Autodesk Inventor part; units mm, degrees
ref_plane "YZ Plane" through (0, 0, 0) normal (1, 0, 0) x (0, 1, 0)
ref_plane "XZ Plane" through (0, 0, 0) normal (0, 1, 0) x (-1, 0, 0)
ref_plane "XY Plane" through (0, 0, 0) normal (0, 0, 1) x (1, 0, 0)
sketch "Sketch1" plane through (0, 0, 0) normal (0, 0, 1) x (1, 0, 0)
  arc A0 (-16, 4) -> (-16, -4) centre (-16, 0) ccw
  arc A1 (16, -4) -> (16, 4) centre (16, 0) ccw
  line L0 (-16, -4) -> (16, -4)
  line L1 (-16, 4) -> (16, 4)
  line L2 (-28, 0) -> (28, 0)
  line L3 (0, -5.6) -> (0, 5.6)
  point P0 (0, 0)
  dimension "d3" = 4
  dimension "d4" = 4
  dimension "d5" = 32
  dimension "d6" = 32
  dimension "d7" = 0
  dimension "d8" = 16
  dimension "d9" = 32
  dimension "d10" = 32
extrude "Extrusion1" add sketch "Sketch1" along normal blind 8
sketch "Sketch2" plane through (0, 0, 8) normal (0, 0, 1) x (1, 0, 0)
  arc A0 (-16, 4) -> (-16, -4) centre (-16, 0) ccw
  circle A1 centre (-16, 0) radius 2.5
  line L0 (-28, 0) -> (28, 0)
  circle A2 centre (-8, 0) radius 2.5
  circle A3 centre (0, 0) radius 2.5
  circle A4 centre (8, 0) radius 2.5
  circle A5 centre (16, 0) radius 2.5
  dimension "d13" = 5
  dimension "d19" = 8
extrude "Extrusion2" cut sketch "Sketch2" against normal through all
sketch "Sketch3" plane through (0, 0, 8) normal (0, 0, 1) x (1, 0, 0)
  circle A0 centre (16, 0) radius 2.5
  circle A1 centre (8, 0) radius 2.5
  circle A2 centre (0, 0) radius 2.5
  circle A3 centre (-8, 0) radius 2.5
  circle A4 centre (-16, 0) radius 2.5
  arc A5 (-16, 4) -> (-16, -4) centre (-16, 0) ccw
  circle A6 centre (-16, 0) radius 3
  line L0 (-28, 0) -> (28, 0)
  circle A7 centre (-8, 0) radius 3
  circle A8 centre (0, 0) radius 3
  circle A9 centre (8, 0) radius 3
  circle A10 centre (16, 0) radius 3
  dimension "d23" = 6
  dimension "d29" = 8
extrude "Extrusion3" cut sketch "Sketch3" against normal blind 0.8 contours L0 A10 A0 | A0 L0 A10 | A6 L0 A4 | L0 A4 A6 | A7 L0 A3 | L0 A3 A7 | A8 L0 A2 | L0 A2 A8 | A9 L0 A1 | L0 A1 A9
sketch "Sketch4" plane through (0, 0, 0) normal (0, 0, -1) x (-1, 0, 0)
  circle A0 centre (-16, 0) radius 2.5
  circle A1 centre (-8, 0) radius 2.5
  circle A2 centre (0, 0) radius 2.5
  circle A3 centre (8, 0) radius 2.5
  circle A4 centre (16, 0) radius 2.5
  arc A5 (-16, 4) -> (-16, -4) centre (-16, 0) ccw
  circle A6 centre (-16, 0) radius 3
  line L0 (28, 0) -> (-28, 0)
  circle A7 centre (-8, 0) radius 3
  circle A8 centre (0, 0) radius 3
  circle A9 centre (8, 0) radius 3
  circle A10 centre (16, 0) radius 3
  dimension "d33" = 6
  dimension "d39" = 8
extrude "Extrusion4" cut sketch "Sketch4" against normal blind 0.8 contours L0 A6 A0 | A0 L0 A6 | A10 L0 A4 | L0 A4 A10 | A9 L0 A3 | L0 A3 A9 | A8 L0 A2 | L0 A2 A8 | A7 L0 A1 | L0 A1 A7
sketch "Sketch5" plane through (0, 0, 8) normal (0, 0, 1) x (1, 0, 0)
  circle A0 centre (-8, 0) radius 3
  arc A1 (-16, 4) -> (-16, -4) centre (-16, 0) ccw
  arc A2 (-14.1972, -3) -> (-14.1972, 3) centre (-16, 0) ccw
  arc A3 (-9.8028, 3) -> (-9.8028, -3) centre (-8, 0) ccw
  line L0 (-14.1972, 3) -> (-9.8028, 3)
  line L1 (-14.1972, -3) -> (-9.8028, -3)
  line L2 (-28, 0) -> (28, 0)
  arc A4 (-6.1972, -3) -> (-6.1972, 3) centre (-8, 0) ccw
  arc A5 (-1.8028, 3) -> (-1.8028, -3) centre (0, 0) ccw
  line L3 (-6.1972, 3) -> (-1.8028, 3)
  line L4 (-6.1972, -3) -> (-1.8028, -3)
  arc A6 (1.8028, -3) -> (1.8028, 3) centre (0, 0) ccw
  arc A7 (6.1972, 3) -> (6.1972, -3) centre (8, 0) ccw
  line L5 (1.8028, 3) -> (6.1972, 3)
  line L6 (1.8028, -3) -> (6.1972, -3)
  arc A8 (9.8028, -3) -> (9.8028, 3) centre (8, 0) ccw
  arc A9 (14.1972, 3) -> (14.1972, -3) centre (16, 0) ccw
  line L7 (9.8028, 3) -> (14.1972, 3)
  line L8 (9.8028, -3) -> (14.1972, -3)
  dimension "d43" = 3.5
  dimension "d44" = 3.5
  dimension "d45" = 4.3944
  dimension "d46" = 4.3944
  dimension "d52" = 8
extrude "Extrusion5" cut sketch "Sketch5" against normal through all contours A3 L1 A2 L2 | L2 A2 L0 A3 | A8 L7 A9 L2 | L2 A9 L8 A8 | A6 L5 A7 L2 | L2 A7 L6 A6 | A4 L3 A5 L2 | L2 A5 L4 A4
properties part number "5M Beam"
Model file for the job. Use its own axes, mm. A direction names the side the tool comes from. Coordinates: 2 decimals unless noted, no trailing zeros. Write each loop counter-clockwise with the first axis right and the second up, starting at its lowest first coordinate (ties: lowest second). Pieces come first, ordered by that corner, then holes. Notation, with made-up numbers: (57.25, 14) - (86.25, 14) arc R22 ccw to (86.25, 44) - close; hole circle Ø6 at (6, 63.25). An arc over 180 degrees is marked (long way). Use a Markdown table: item, result. Add a question column.
Item 1: Two-plate mould, pull along Y, no slides. Class faces 4 (the face through (-3, -1, 0)), 5 (the face through (-20, 0, 4)), 6 (the face through (-3, 0.1, 7.6)): pulls with the +Y half, pulls with the -Y half, needs draft (parallel to the pull), parting line crosses it, or undercut.
Item 2: 3-axis set-ups, long thin cutter, end or side, ignore diameter. For faces 1 (the face through (-0.54, -2.44, 4.04)), 2 (the face through (-13, 0.1, 0.4)), 3 (the face through (-19, 0.1, 7.6)): which of +Z, -Z, +X, -X, +Y, -Y reach the whole face in a straight line?
Item 3: Band-saw the part on B-B, the plane x = 8. Write the cut outline in (y, z), and give its area (3 significant figures).
Item 4: Drill centre lines: line 1 along Y through (x, z) = (-5, 5.5); line 2 along Y through (x, z) = (-12, 3.75); line 3 along Y through (x, z) = (16, 6). Where is each one in solid material? Low to high.
Item 5: Drop flat-ended pins along their axis: pin 1 (4.5 mm diameter, centred on x = 0, y = 0, fed in from +Z); pin 2 (1.5 mm diameter, centred on y = -1, z = 1.5, fed in from +X); pin 3 (1.5 mm diameter, centred on y = -2.5, z = 4, fed in from -X); pin 4 (4 mm diameter, centred on y = 3, z = 4.5, fed in from -X). Give the stop position or say it passes through.
Item 6: Band-saw the part on A-A, the plane z = 1.5. Give the number of separate pieces and of enclosed holes in the cut face, and give its area (3 significant figures).
A:
| question | item | result |
|---|---|---|
| 1 | face 4 | needs draft |
| 1 | face 5 | parting line crosses it |
| 1 | face 6 | undercut |
| 2 | face 1 | +Z, -Z |
| 2 | face 2 | -Z |
| 2 | face 3 | +Z |
| 3 | outline | (-4, 0) - (-3, 0) - (-3, 0.8) - (-2.5, 0.8) - (-2.5, 7.2) - (-3, 7.2) - (-3, 8) - (-4, 8) - close; (2.5, 0.8) - (3, 0.8) - (3, 0) - (4, 0) - (4, 8) - (3, 8) - (3, 7.2) - (2.5, 7.2) - close |
| 3 | area | 22.4 mm² |
| 4 | line 1 | y = -4 to -3, -1.8 to 1.8, 3 to 4 |
| 4 | line 2 | y = -4 to -3, 3 to 4 |
| 4 | line 3 | y = -4 to -2.5, 2.5 to 4 |
| 5 | pin 1 | passes through |
| 5 | pin 2 | stops at x = 19.99 |
| 5 | pin 3 | stops at x = -19.6 |
| 5 | pin 4 | stops at x = -19.87 |
| 6 | separate pieces | 1 |
| 6 | enclosed holes | 9 |
| 6 | area | 160 mm² |
